```python
from build123d import *

# Parameters (mm, degrees)
SKETCH2_R           = 2.5
SKETCH2_R_2         = 2
BOSS_EXTRUDE1_DEPTH = 10
SKETCH4_R           = 1.5
CUT_EXTRUDE3_DEPTH  = 16
SKETCH7_R           = 10
BOSS_EXTRUDE4_DEPTH = 10
SKETCH8_R           = 1.55
SKETCH8_R_2         = 3.5
CUT_EXTRUDE7_DEPTH  = 10


with BuildPart() as part:
    # Sketch2 → Boss-Extrude1 (new body)
    with BuildSketch(Plane(origin=(0, 0, 0), x_dir=(1, 0, 0), z_dir=(0, 1, 0))):
        with BuildLine():
            Line((0, 7.5), (100, 7.5))
            ThreePointArc((100, 7.5), (107.5, 0), (100, -7.5))
            Line((100, -7.5), (0, -7.5))
            ThreePointArc((0, -7.5), (-7.5, 0), (0, 7.5))
        make_face()
        Circle(SKETCH2_R, mode=Mode.SUBTRACT)
        with Locations((100, 0)):
            Circle(SKETCH2_R_2, mode=Mode.SUBTRACT)
    extrude(amount=BOSS_EXTRUDE1_DEPTH)

    # Sketch4 → Cut-Extrude3 (cut, through all)
    with BuildSketch(Plane(origin=(0, 0, -7.5), x_dir=(-1, 0, 0), z_dir=(0, 0, -1))):
        with Locations((0, 5)):
            Circle(SKETCH4_R)
    extrude(amount=-CUT_EXTRUDE3_DEPTH, mode=Mode.SUBTRACT)

    # Sketch7 → Boss-Extrude4 (add)
    with BuildSketch(Plane(origin=(0, 10, 0), x_dir=(1, 0, 0), z_dir=(0, 1, 0))):
        Circle(SKETCH7_R)
    extrude(amount=-BOSS_EXTRUDE4_DEPTH)

    # Sketch8 → Cut-Extrude7 (cut)
    with BuildSketch(Plane(origin=(0, 10, 0), x_dir=(1, 0, 0), z_dir=(0, 1, 0))):
        with Locations((0, 7)):
            Circle(SKETCH8_R)
        with Locations((7, 0)):
            Circle(SKETCH8_R)
        with Locations((0, -7)):
            Circle(SKETCH8_R)
        with Locations((-7, 0)):
            Circle(SKETCH8_R)
        Circle(SKETCH8_R_2)
    extrude(amount=-CUT_EXTRUDE7_DEPTH, mode=Mode.SUBTRACT)


solid = part.part
```
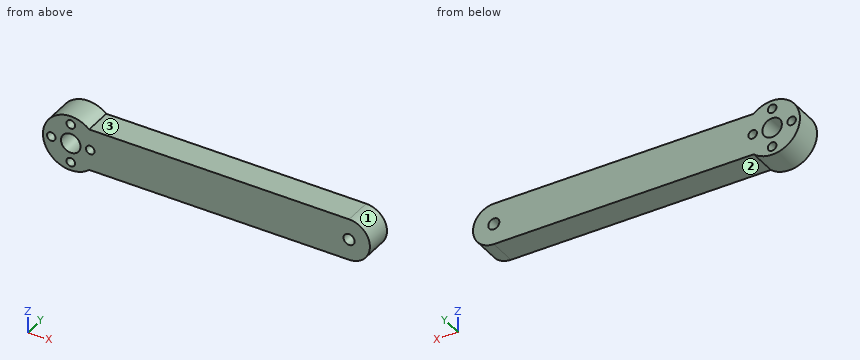
Geometry: final body of the model. Coordinates: model frame, mm. Face numbers are marked on the shaded views. A direction names the side the tool comes from. Round coordinates to 2 decimals unless told otherwise and drop trailing zeros. Write each loop counter-clockwise with the first axis right and the second up, starting at its lowest first coordinate (ties: lowest second). Pieces come first, ordered by that corner, then holes.
Item 1: Pin query (flat end, axial travel): P1, Ø5, axis at x = 25, y = 4, coming from the +Z side; P2, Ø3, axis at x = 0, z = 7, coming from the +Y side; P3, Ø5, axis at x = 72.5, y = 3.5, coming from the -Z side; P4, Ø5, axis at x = 7, y = 3.5, coming from the +Z side. Return the tip coordinate at first contact, or that it passes through.
Item 2: Section query B-B (y = 2.25). Return loops of the section in (x, z).
Item 3: Set-up query: the marked faces 1, 2 and 3. Return all of +Z, -Z, +X, -X, +Y, -Y with unobstructed straight access to the full face (end or side cutting, diameter ignored); none if empty.
Item 4: Section query C-C (x = 40). Return loops of the section in (y, z), plus the area to 3 significant figures.
Item 5: Section query A-A (z = 0). Return loops of the section in (x, y), plus the area to 3 significant figures.
Item 6: Material intervals for L1, parallel to Z at x = 0, y = 4.5; L2, parallel to Z at x = 100, y = 7.25; L3, parallel to Z at x = 7, y = 5, sorted ascending.
Completed:
1. P1: stops at z = 7.5
1. P2: passes through
1. P3: stops at z = -7.5
1. P4: stops at z = 8.93
2. outline: (6.61, -7.5) - (100, -7.5) arc R7.5 ccw to (100, 7.5) - (6.61, 7.5) arc R10 ccw (long way) to start; hole circle Ø3.1 at (-7, 0); hole circle Ø7 at (0, 0); hole circle Ø3.1 at (0, -7); hole circle Ø3.1 at (0, 7); hole circle Ø3.1 at (7, 0); hole circle Ø4 at (100, 0)
3. face 1: +X, +Y, -Y
3. face 2: -Z, +X, +Y, -Y
3. face 3: +Z, +X, +Y, -Y
4. outline: (0, -7.5) - (10, -7.5) - (10, 7.5) - (0, 7.5) - close
4. area: 150 mm2
5. outline: (-10, 0) - (-8.55, 0) - (-8.55, 10) - (-10, 10) - close; (-5.45, 0) - (-3.5, 0) - (-3.5, 10) - (-5.45, 10) - close; (3.5, 0) - (5.45, 0) - (5.45, 10) - (3.5, 10) - close; (8.55, 0) - (98, 0) - (98, 10) - (8.55, 10) - close; (102, 0) - (107.5, 0) - (107.5, 10) - (102, 10) - close
5. area: 1,000 mm2
6. L1: z = -10 to -8.55, -5.45 to -3.5, 3.5 to 5.45, 8.55 to 10
6. L2: z = -7.5 to -2, 2 to 7.5
6. L3: z = -7.5 to -1.55, 1.55 to 7.5
